```python
from build123d import *

# Parameters (mm, degrees)
SKETCH1_W           = 178
SKETCH1_H           = 120
SKETCH1_R           = 19.05
SKETCH1_R_2         = 7.15
SKETCH1_W_2         = 138.4
SKETCH1_H_2         = 9.9
BOSS_EXTRUDE1_DEPTH = 9.5
M4_TAPPED_HOLE1_D   = 3.3
M5_TAPPED_HOLE1_D   = 4.2


with BuildPart() as part:
    # Sketch1 → Boss-Extrude1 (new body)
    with BuildSketch(Plane(origin=(0, 0, 0), x_dir=(1, 0, 0), z_dir=(0, 1, 0))):
        Rectangle(SKETCH1_W, SKETCH1_H)
        with Locations((0, -28)):
            Circle(SKETCH1_R, mode=Mode.SUBTRACT)
        with Locations((-59, -24)):
            Circle(SKETCH1_R_2, mode=Mode.SUBTRACT)
        with Locations((59, -24)):
            Circle(SKETCH1_R_2, mode=Mode.SUBTRACT)
        with Locations((0, 44.95)):
            Rectangle(SKETCH1_W_2, SKETCH1_H_2, mode=Mode.SUBTRACT)
    extrude(amount=BOSS_EXTRUDE1_DEPTH)

    # M4 Tapped Hole1 (through all)
    with Locations(Plane(origin=(0, 9.5, 0), x_dir=(1, 0, 0), z_dir=(0, 1, 0))):
        with Locations((-80.25, 28), (0, 28), (80.25, 28)):
            Hole(M4_TAPPED_HOLE1_D / 2)

    # M5 Tapped Hole1 (through all)
    with Locations(Plane(origin=(0, 9.5, 0), x_dir=(1, 0, 0), z_dir=(0, 1, 0))):
        with Locations((-23.55, -4.45), (23.55, -4.45), (23.55, -51.55), (-23.55, -51.55)):
            Hole(M5_TAPPED_HOLE1_D / 2)


solid = part.part
```
Design review of the part built by this model. Coordinates are the model's own, in mm. A direction names the side the tool comes from. Give positions to 0.01 mm unless a question says otherwise; leave off trailing zeros. Order: outer loops, then holes, each group sorted by start corner. A loop starts at its lowest first (then second) coordinate and runs counter-clockwise, first axis right, second up. Notation, with made-up numbers: (25.25, 49.5) - (64.25, 49.5) arc R20 cw to (64.25, 68.5) - close; hole circle Ø3 at (18.5, 37). An arc over 180 degrees is marked (long way). Use a Markdown table: item, result. Add a question column.
(1) Add section A-A on x = 59. Give the boundary of the cut face in (y, z), then the cut area to 3 significant figures.
(2) Mouldability with a two-part tool opening along Z and no side actions: class faces 3 (the face through (89, 5, 1)), 4 (the face through (-69.2, 5, -45)), 5 (the face through (-21.45, 4.68, 4.36)), 6 (the face through (-1, 5, -60)) as +Z half, -Z half, draft (parallel to the pull), parting line (faces both ways), or undercut.
(3) Wall thickness on probe 1 along Z at (x, y) = (59, 6); probe 2 along X at (y, z) = (5, -28); probe 3 along Z at (x, y) = (-40.5, 0.5): over which ranges is each line inside the solid? List them lowest first. Write a range as [from, to].
(4) Add section D-D on x = -48. Give the boundary of the cut face in (y, z), then the cut area to 3 significant figures.
(5) Add section C-C on y = 2. Give the number of separate pieces and of enclosed holes in the cut face, then the cut area to 3 significant figures.
(6) Add section B-B on z = 51.55. Give the boundary of the cut face in (x, y), then the cut area to 3 significant figures.
(7) Machinability: for faces 1 (the face through (-1, 5, 60)), 2 (the face through (69.2, 5, -45)), which of the approach directions +Z, -Z, +X, -X, +Y, -Y give a long, thin tool a straight path to every point of the face, cutting with its end or side? Answer none if there is none.
(8) Clearance check with a flat-ended pin moving along its axis: P1, Ø8.5, axis at x = 59, z = 24, coming from the +Y side. State where the tip first meets the part, or that it passes through.
Report:
| question | item | result |
|---|---|---|
| 1 | outline | (0, -60) - (9.5, -60) - (9.5, -49.9) - (0, -49.9) - close; (0, -40) - (9.5, -40) - (9.5, 16.85) - (0, 16.85) - close; (0, 31.15) - (9.5, 31.15) - (9.5, 60) - (0, 60) - close |
| 1 | area | 910 mm² |
| 2 | face 3 | draft |
| 2 | face 4 | undercut |
| 2 | face 5 | undercut |
| 2 | face 6 | -Z half |
| 3 | probe 1 | z = [-60, -49.9], [-40, 16.85], [31.15, 60] |
| 3 | probe 2 | x = [-89, -81.9], [-78.6, -1.65], [1.65, 78.6], [81.9, 89] |
| 3 | probe 3 | z = [-60, -49.9], [-40, 60] |
| 4 | outline | (0, -60) - (9.5, -60) - (9.5, -49.9) - (0, -49.9) - close; (0, -40) - (9.5, -40) - (9.5, 60) - (0, 60) - close |
| 4 | area | 1,050 mm² |
| 5 | separate pieces | 1 |
| 5 | enclosed holes | 11 |
| 5 | area | 18,400 mm² |
| 6 | outline | (-89, 0) - (-25.65, 0) - (-25.65, 9.5) - (-89, 9.5) - close; (-21.45, 0) - (21.45, 0) - (21.45, 9.5) - (-21.45, 9.5) - close; (25.65, 0) - (89, 0) - (89, 9.5) - (25.65, 9.5) - close |
| 6 | area | 1,610 mm² |
| 7 | face 1 | +Z, +X, -X, +Y, -Y |
| 7 | face 2 | +Y, -Y |
| 8 | P1 | passes through |
